Read the model definition and answer for the solid it produces. Units are mm, in the model's axes. A direction names the side the tool comes from. Coordinates: 2 decimals unless noted, no trailing zeros. Loops run counter-clockwise (first coordinate to the right, second up) from the corner with the lowest first, then second, coordinate; pieces in that order, holes last. Notation, with made-up numbers: M -40,-34 L -27,-34 A23 ccw -27,-9 Z; hole C 22.5,57 d6. An arc over 180 degrees is marked long. One line per item, written item: value. Start each with the question number.
1. Determine the mould class of faces 1 (the face through (1.717, 0.541, 5.57)), 2 (the face through (0, 0, 0)), 3 (the face through (-0.338, 2.578, 5.43)) for opening direction Y: +Y half, -Y half, draft (parallel to the pull), parting line (faces both ways), or undercut.
2. The part is cut by section C-C (z = 2.25). Write down the section's boundary in (x, y).
3. Consider probe 1 along Y at (x, z) = (0, 4.5); probe 2 along Z at (x, y) = (-0.75, -3.5); probe 3 along Y at (x, z) = (-1, 8.75). Determine where each line is inside the solid, lowest interval first.
4. For faces 4 (the face through (2, 1, 10.5)), 5 (the face through (0, 0, 0.5)), determine the directions among +Z, -Z, +X, -X, +Y, -Y from which every point of the face is accessible in a straight line to the end or side of a thin tool.
5. The part is cut by section D-D (x = 2). Write down the section's boundary in (y, z), then the cut area to 3 significant figures.
6. The part is cut by section A-A (x = 0). Write down the section's boundary in (y, z).
7. Flat-ended cylindrical pins translate along their axes: pin 1 (1.8 mm diameter, centred on x = 0.5, y = -0.5, fed in from +Z); pin 2 (2 mm diameter, centred on x = -2, y = 1, fed in from -Z); pin 3 (4 mm diameter, centred on x = 2.5, z = 3, fed in from +Y). Find the tip coordinate at first contact, or state that the pin passes through.
```python
from build123d import *

# Parameters (mm, degrees)
SKETCH1_W           = 8
SKETCH1_H           = 8
BOSS_EXTRUDE1_DEPTH = 0.5
SKETCH4_R           = 2.6
BOSS_EXTRUDE3_DEPTH = 10
SKETCH6_R           = 1.8
CUT_EXTRUDE2_DEPTH  = 10


with BuildPart() as part:
    # Sketch1 → Boss-Extrude1 (new body)
    with BuildSketch(Plane.XY):
        Rectangle(SKETCH1_W, SKETCH1_H)
    extrude(amount=BOSS_EXTRUDE1_DEPTH)

    # Sketch4 → Boss-Extrude3 (add)
    with BuildSketch(Plane.XY.offset(0.5)):
        Circle(SKETCH4_R)
    extrude(amount=BOSS_EXTRUDE3_DEPTH)

    # Sketch6 → Cut-Extrude2 (cut)
    with BuildSketch(Plane.XY.offset(10.5)):
        Circle(SKETCH6_R)
    extrude(amount=-CUT_EXTRUDE2_DEPTH, mode=Mode.SUBTRACT)


solid = part.part
```
Answer block:
1. face 1: undercut
1. face 2: draft
1. face 3: parting line
2. outline: C 0,0 d5.2; hole C 0,0 d3.6
3. probe 1: y = -2.6 to -1.8, 1.8 to 2.6
3. probe 2: z = 0 to 0.5
3. probe 3: y = -2.4 to -1.5, 1.5 to 2.4
4. face 4: +Z, +X, -X, +Y, -Y
4. face 5: +Z
5. outline: M -4,0 L 4,0 L 4,0.5 L 1.66,0.5 L 1.66,10.5 L -1.66,10.5 L -1.66,0.5 L -4,0.5 Z
5. area: 37.2 mm2
6. outline: M -4,0 L 4,0 L 4,0.5 L 2.6,0.5 L 2.6,10.5 L 1.8,10.5 L 1.8,0.5 L -1.8,0.5 L -1.8,10.5 L -2.6,10.5 L -2.6,0.5 L -4,0.5 Z
7. pin 1: stops at z = 0.5
7. pin 2: stops at z = 0
7. pin 3: stops at y = 2.55
